CAD build for the part. Positions are in the model's coordinates, mm. Face numbers are marked on the shaded views. Coordinates: 2 decimals unless noted, no trailing zeros. Loops run counter-clockwise (first coordinate to the right, second up) from the corner with the lowest first, then second, coordinate; pieces in that order, holes last. Notation, with made-up numbers: (-13, 59.25) -> (5, 59.25) arc R17 cw to (5, 80.25) -> close; hole circle Ø11 at (-11.5, 23.25). An arc over 180 degrees is marked (long way). Answer as CSV lines item,"result". Start each with the question number.
```python
from build123d import *

# Parameters (mm, degrees)
SKETCH1_R                   = 9.525
BOSS_EXTRUDE1_DEPTH         = 5.08
F_43_0_089_DIAMETER_HOLE1_D = 2.2606
CIRPATTERN1_COUNT           = 4


with BuildPart() as part:
    # Sketch1 → Boss-Extrude1 (new body)
    with BuildSketch(Plane(origin=(0, 0, 0), x_dir=(1, 0, 0), z_dir=(0, 1, 0))):
        Circle(SKETCH1_R)
        with BuildLine():
            Line((0.624652949, -2.420704173), (2.420704173, -0.624652949))
            ThreePointArc((2.420704173, -0.624652949), (-1.767766953, 1.767766953), (0.624652949, -2.420704173))
        make_face(mode=Mode.SUBTRACT)
    extrude(amount=BOSS_EXTRUDE1_DEPTH)

    # #43 (0.089) Diameter Hole1 (through all)
    with Locations(Plane(origin=(0, 5.08, 0), x_dir=(1, 0, 0), z_dir=(0, 1, 0))):
        with Locations((0, 6.413072646)):
            f_43_0_089_diameter_hole1 = Hole(F_43_0_089_DIAMETER_HOLE1_D / 2)

    # CirPattern1: #43 (0.089) Diameter Hole1 ×4 about axis
    cirpattern1_axis = Axis((0, 0, 0), (0, 1, 0))
    for i in range(1, CIRPATTERN1_COUNT):
        add(f_43_0_089_diameter_hole1.rotate(cirpattern1_axis, i * 360 / CIRPATTERN1_COUNT), mode=Mode.SUBTRACT)


solid = part.part
```
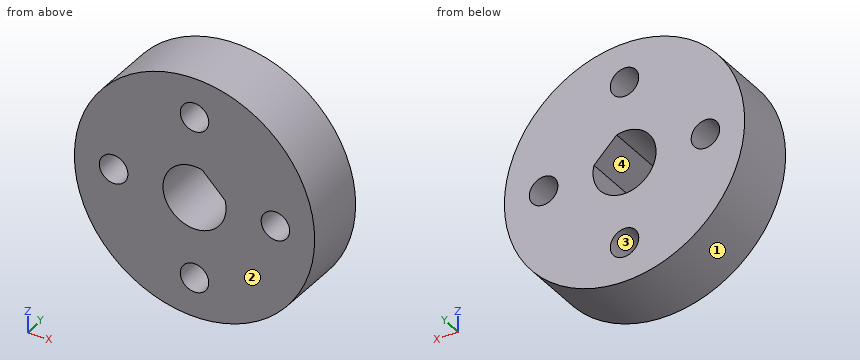
Q1. Pin check, flat tips, straight feed: pin 1 Ø3 at (x, z) = (-6.41, 0) entering from +Y; pin 2 Ø1.5 at (y, z) = (4.5, 7) entering from +X; pin 3 Ø3 at (y, z) = (2.5, 7) entering from +X. Stop position of each tip, or through.
Q2. Saw through at A-A (x = 0). List the corners of the cut face in (y, z) (3 decimals).
Q3. Saw through at B-B (z = 0). List the corners of the cut face in (x, y) (3 decimals), and give its area (3 significant figures).
Q4. Saw through at D-D (y = 2.9). List the corners of the cut face in (x, z) (3 decimals), and give its area (3 significant figures).
Q5. Probe probe 1 along X at (y, z) = (3.1, 0) (3 decimals); probe 2 along X at (y, z) = (1.3, -0.75). List the from-to ranges inside material, lowest first. Write a range as from..to.
Q6. Saw through at C-C (x = -6). List the corners of the cut face in (y, z), and give its area (3 significant figures).
Q7. Two-plate mould, pull along X, no slides. Class the marked faces 1, 2, 3 and 4: pulls with the +X half, pulls with the -X half, needs draft (parallel to the pull), parting line crosses it, or undercut.
Ans:
1,pin 1,"stops at y = 5.08"
1,pin 2,"stops at x = 7.19"
1,pin 3,"stops at x = 7.78"
2,outline,"(0, -9.525) -> (5.08, -9.525) -> (5.08, -7.543) -> (0, -7.543) -> close; (0, -5.283) -> (5.08, -5.283) -> (5.08, -2.5) -> (0, -2.5) -> close; (0, 2.5) -> (5.08, 2.5) -> (5.08, 5.283) -> (0, 5.283) -> close; (0, 7.543) -> (5.08, 7.543) -> (5.08, 9.525) -> (0, 9.525) -> close"
3,outline,"(-9.525, 0) -> (-7.543, 0) -> (-7.543, 5.08) -> (-9.525, 5.08) -> close; (-5.283, 0) -> (-2.5, 0) -> (-2.5, 5.08) -> (-5.283, 5.08) -> close; (2.5, 0) -> (5.283, 0) -> (5.283, 5.08) -> (2.5, 5.08) -> close; (7.543, 0) -> (9.525, 0) -> (9.525, 5.08) -> (7.543, 5.08) -> close"
3,area,"48.4 mm²"
4,outline,"circle Ø19.05 at (0, 0); hole circle Ø2.261 at (-6.413, 0); hole circle Ø2.261 at (0, -6.413); hole circle Ø2.261 at (0, 6.413); hole (0.625, 2.421) arc R2.5 ccw (long way) to (2.421, 0.625) -> close; hole circle Ø2.261 at (6.413, 0)"
4,area,"250 mm²"
5,probe 1,"x = -9.525..-7.543, -5.283..-2.5, 2.5..5.283, 7.543..9.525"
5,probe 2,"x = -9.5..-7.26, -5.57..-2.38, 2.38..5.57, 7.26..9.5"
6,outline,"(0, -7.4) -> (5.08, -7.4) -> (5.08, -1.05) -> (0, -1.05) -> close; (0, 1.05) -> (5.08, 1.05) -> (5.08, 7.4) -> (0, 7.4) -> close"
6,area,"64.5 mm²"
7,face 1,"parting line crosses it"
7,face 2,"needs draft"
7,face 3,"undercut"
7,face 4,"undercut"
